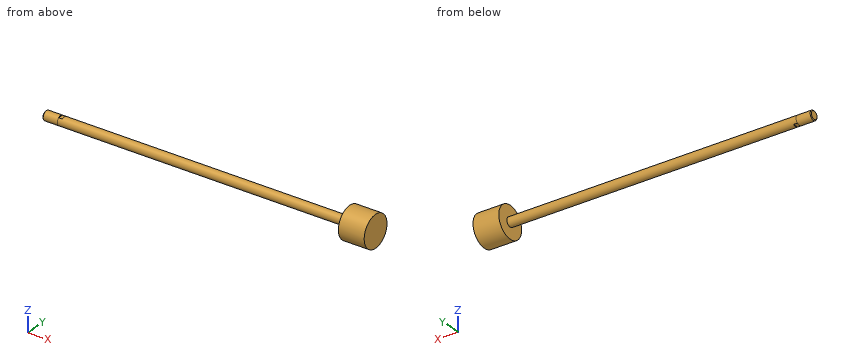
Autodesk Inventor part; units mm, degrees
ref_plane "dia1_XY" through (-3.175, 3.9624, 0) normal (1, 0, 0) x (0, 0, -1)
ref_plane "dia1_YZ" through (-3.175, 3.9624, 0) normal (0, 0, -1) x (0, 1, 0)
ref_plane "dia1_ZX" through (-3.175, 3.9624, 0) normal (0, 1, 0) x (1, 0, 0)
sketch "Sketch_1" plane through (0, 0, 0) normal (0, 0, 1) x (1, 0, 0)
  line L0 (266.5984, 0) -> (-3.175, 0)
  line L1 (-3.175, 0) -> (-3.175, 3.9624)
  line L2 (-3.175, 3.9624) -> (244.475, 3.9624)
  line L3 (244.475, 3.9624) -> (244.475, 13.5572)
  line L4 (244.475, 13.5572) -> (266.5984, 13.5572)
  line L5 (266.5984, 13.5572) -> (266.5984, 0)
  line L6 (266.5984, 0) -> (-3.175, 0)
revolve "Revolution1" add sketch "Sketch_1" angle 360 about axis through (266.5984, 0, 0) along (1, 0, 0)
sketch "Sketch_3" plane through (0, 0, 0) normal (0, 0, 1) x (1, 0, 0)
  line L0 (-3.175, 0) -> (-15.875, 0)
  line L1 (-15.875, 0) -> (-15.875, 3.3388)
  line L2 (-15.875, 3.3388) -> (-15.2451, 3.9688)
  line L3 (-15.2451, 3.9688) -> (-3.175, 3.9688)
  line L4 (-3.175, 3.9688) -> (-3.175, 0)
  line L5 (-3.175, 0) -> (-15.875, 0)
revolve "Revolution2" add sketch "Sketch_3" angle 360 about axis through (-3.175, 0, 0) along (1, 0, 0)
thread "Thread1"
sketch "Sketch_10" plane through (-3.175, 0, 0) normal (1, 0, 0) x (0, 0, -1)
  line L0 (-7.9248, 7.9248) -> (-7.9248, -7.9248)
  line L1 (-7.9248, -7.9248) -> (7.9248, -7.9248)
  line L2 (7.9248, -7.9248) -> (7.9248, 7.9248)
  line L3 (7.9248, 7.9248) -> (-7.9248, 7.9248)
  line L4 (-3.175, 3.9624) -> (-3.175, -3.9624)
  line L5 (-3.175, -3.9624) -> (3.175, -3.9624)
  line L6 (3.175, -3.9624) -> (3.175, 3.9624)
  line L7 (3.175, 3.9624) -> (-3.175, 3.9624)
extrude "Extrusion1" cut sketch "Sketch_10" along normal blind 3.175
ref_plane "dia1_XY" through (-3.175, 3.9624, 0) normal (1, 0, 0) x (0, 0, -1)
ref_plane "dia1_YZ" through (-3.175, 3.9624, 0) normal (0, 0, -1) x (0, 1, 0)
ref_plane "dia1_ZX" through (-3.175, 3.9624, 0) normal (0, 1, 0) x (1, 0, 0)
ref_plane "dia12_XY" through (0, 0, 14.1351) normal (1, 0, 0) x (0, 0, -1)
ref_plane "dia12_YZ" through (0, 0, 14.1351) normal (0, 0, -1) x (0, 1, 0)
ref_plane "dia12_ZX" through (0, 0, 14.1351) normal (0, 1, 0) x (1, 0, 0)
ref_plane "dia2_XY" through (-3.175, -3.9624, 0) normal (1, 0, 0) x (0, 0, -1)
ref_plane "dia2_YZ" through (-3.175, -3.9624, 0) normal (0, 0, -1) x (0, 1, 0)
ref_plane "dia2_ZX" through (-3.175, -3.9624, 0) normal (0, 1, 0) x (1, 0, 0)
ref_plane "dia22_XY" through (0, 0, -14.1351) normal (1, 0, 0) x (0, 0, -1)
ref_plane "dia22_YZ" through (0, 0, -14.1351) normal (0, 0, -1) x (0, 1, 0)
ref_plane "dia22_ZX" through (0, 0, -14.1351) normal (0, 1, 0) x (1, 0, 0)
ref_plane "rl1_XY" through (-15.875, 0, 0) normal (1, 0, 0) x (0, 0, -1)
ref_plane "rl1_YZ" through (-15.875, 0, 0) normal (0, 0, -1) x (0, 1, 0)
ref_plane "rl1_ZX" through (-15.875, 0, 0) normal (0, 1, 0) x (1, 0, 0)
ref_plane "rl2_XY" through (-3.175, 0, 0) normal (1, 0, 0) x (0, 0, -1)
ref_plane "rl2_YZ" through (-3.175, 0, 0) normal (0, 0, -1) x (0, 1, 0)
ref_plane "rl2_ZX" through (-3.175, 0, 0) normal (0, 1, 0) x (1, 0, 0)
ref_plane "rod_cp_XY" through (0, 0, 0) normal (1, 0, 0) x (0, 0, -1)
ref_plane "rod_cp_YZ" through (0, 0, 0) normal (0, 0, -1) x (0, 1, 0)
ref_plane "rod_cp_ZX" through (0, 0, 0) normal (0, 1, 0) x (1, 0, 0)
ref_plane "thd1_XY" through (-15.875, 3.9688, 0) normal (1, 0, 0) x (0, 0, -1)
ref_plane "thd1_YZ" through (-15.875, 3.9688, 0) normal (0, 0, -1) x (0, 1, 0)
ref_plane "thd1_ZX" through (-15.875, 3.9688, 0) normal (0, 1, 0) x (1, 0, 0)
ref_plane "thd2_XY" through (-15.875, -3.9688, 0) normal (1, 0, 0) x (0, 0, -1)
ref_plane "thd2_YZ" through (-15.875, -3.9688, 0) normal (0, 0, -1) x (0, 1, 0)
ref_plane "thd2_ZX" through (-15.875, -3.9688, 0) normal (0, 1, 0) x (1, 0, 0)
ref_plane "to_rod_clevis_XY" through (-20.701, 0, 0) normal (1, 0, 0) x (0, 0, -1)
ref_plane "to_rod_clevis_YZ" through (-20.701, 0, 0) normal (0, 0, -1) x (0, 1, 0)
ref_plane "to_rod_clevis_ZX" through (-20.701, 0, 0) normal (0, 1, 0) x (1, 0, 0)
ref_plane "wf1_XY" through (-3.175, 0, 0) normal (1, 0, 0) x (0, 0, -1)
ref_plane "wf1_YZ" through (-3.175, 0, 0) normal (0, 0, -1) x (0, 1, 0)
ref_plane "wf1_ZX" through (-3.175, 0, 0) normal (0, 1, 0) x (1, 0, 0)
ref_plane "wf2_XY" through (0, 0, 0) normal (1, 0, 0) x (0, 0, -1)
ref_plane "wf2_YZ" through (0, 0, 0) normal (0, 0, -1) x (0, 1, 0)
ref_plane "wf2_ZX" through (0, 0, 0) normal (0, 1, 0) x (1, 0, 0)
ref_plane "wfw1_XY" through (-3.175, 0, -3.175) normal (0, 1, 0) x (1, 0, 0)
ref_plane "wfw1_YZ" through (-3.175, 0, -3.175) normal (1, 0, 0) x (0, 0, -1)
ref_plane "wfw1_ZX" through (-3.175, 0, -3.175) normal (0, 0, -1) x (0, 1, 0)
ref_plane "wfw2_XY" through (-3.175, 0, 3.175) normal (0, 1, 0) x (1, 0, 0)
ref_plane "wfw2_YZ" through (-3.175, 0, 3.175) normal (1, 0, 0) x (0, 0, -1)
ref_plane "wfw2_ZX" through (-3.175, 0, 3.175) normal (0, 0, -1) x (0, 1, 0)
properties part number "C-098-DP0_rod"
Can you work these out from the model? Positions are in its coordinate system, mm. Round coordinates to 2 decimals unless told otherwise and drop trailing zeros. Loops run counter-clockwise (first coordinate to the right, second up) from the corner with the lowest first, then second, coordinate; pieces in that order, holes last. Notation, with made-up numbers: M 72.5,-28 L 79.5,-28 A26 cw 79.5,7 Z; hole C 85.25,-40 d7. An arc over 180 degrees is marked long. Answer in a Markdown table with one row per item.
1. If we section it at A-A, the plane y = 0: Please give me the cut outline in (x, z) (3 decimals).
Established:
| item | result |
|---|---|
| outline | M -15.875,-3.339 L -15.245,-3.969 L -3.175,-3.969 L -3.175,-3.175 L 0,-3.175 L 0,-3.962 L 244.475,-3.962 L 244.475,-13.557 L 266.598,-13.557 L 266.598,13.557 L 244.475,13.557 L 244.475,3.962 L 0,3.962 L 0,3.175 L -3.175,3.175 L -3.175,3.969 L -15.245,3.969 L -15.875,3.339 Z |
2. Please list where these lines run through material, in increasing order: line 1 (X direction, y = 10.75, z = -2.75) (3 decimals); line 2 (Y direction, x = 250, z = 2.25); line 3 (Z direction, x = 201.5, y = -1). Write a range as from..to.
Established:
| item | result |
|---|---|
| line 1 | 244.475..266.598 |
| line 2 | -13.37..13.37 |
| line 3 | -3.83..3.83 |
3. If we section it at C-C, the plane x = 64: Please give me the cut outline in (y, z).
Established:
| item | result |
|---|---|
| outline | C 0,0 d7.92 |
4. If we section it at D-D, the plane y = 10.75: Please give me the cut outline in (x, z) (3 decimals).
Established:
| item | result |
|---|---|
| outline | M 244.475,-8.26 L 266.598,-8.26 L 266.598,8.26 L 244.475,8.26 Z |
5. If we section it at B-B, the plane z = 0: Please give me the cut outline in (x, y) (3 decimals).
Established:
| item | result |
|---|---|
| outline | M -15.875,-3.339 L -15.245,-3.969 L -3.175,-3.969 L -3.175,-3.962 L 244.475,-3.962 L 244.475,-13.557 L 266.598,-13.557 L 266.598,13.557 L 244.475,13.557 L 244.475,3.962 L -3.175,3.962 L -3.175,3.969 L -15.245,3.969 L -15.875,3.339 Z |
6. I'm going to push flat-ended pins straight in: pin 1 Ø10 at (y, z) = (-6.5, 7) entering from -X (3 decimals); pin 2 Ø2.5 at (x, y) = (-1.5, -1) entering from -Z (3 decimals); pin 3 Ø4 at (x, y) = (148, 3.5) entering from +Z. Where does each tip first touch, or does it pass through?
Established:
| item | result |
|---|---|
| pin 1 | x = 244.475 |
| pin 2 | z = -3.175 |
| pin 3 | z = 3.67 |
